Work out the finished part from the listing and answer in its coordinate system (mm). A direction names the side the tool comes from. Give positions to 0.01 mm unless a question says otherwise; leave off trailing zeros. Order: outer loops, then holes, each group sorted by start corner. A loop starts at its lowest first (then second) coordinate and runs counter-clockwise, first axis right, second up.
```python
from build123d import *

# Parameters (mm, degrees)
F0_R          = 25
F1_DEPTH      = 372
F2_R          = 5
F4_DEPTH      = 25
F4_DEPTH_BACK = 397


with BuildPart() as f1:
    # F0 (on Front) → F1 (new body)
    with BuildSketch(Plane.XZ):
        Circle(F0_R)
    extrude(amount=F1_DEPTH)

    # F2
    f2_edges = [f1.edges().sort_by_distance(p)[0] for p in [
        (-25, -372, 0),
        (-25, 0, 0),
    ]]
    fillet(f2_edges, radius=F2_R)

    # F3 (on face) → F4 (join, two sides)
    with BuildSketch(Plane(origin=(0, 0, 0), x_dir=(-1, 0, 0), z_dir=(0, 1, 0))) as f4_sk:
        Polygon((-0.001922, -6), (5.195191, -3.001664), (5.197113, 2.998336), (0.001922, 6), (-5.195191, 3.001664), (-5.197113, -2.998336), align=None)
    extrude(amount=F4_DEPTH)
    extrude(f4_sk.sketch, amount=-F4_DEPTH_BACK)


solid = f1.part
```
1. Straight lines are drawn through the part: probe 1 along X at (y, z) = (-31.5, 1.5); probe 2 along Y at (x, z) = (14, -12); probe 3 along Z at (x, y) = (1, -219.5). For each, find the intervals that lie inside material, in ascending order.
Findings below:
probe 1: x = -24.95 to 24.95
probe 2: y = -372 to 0
probe 3: z = -24.98 to 24.98
2. Which of the six approach directions +Z, -Z, +X, -X, +Y, -Y give full straight-line access (tool end or side, diameter ignored) to faces 1 (the face through (0, 25, 0)), 2 (the face through (4, -372, -4)), 3 (the face through (4, 0, -4))?
Findings below:
face 1: +Z, -Z, +X, -X, +Y
face 2: -Y
face 3: +Y
3. The part is cut by section A-A (y = -319). Write down the section's boundary in (x, z).
Findings below:
outline: circle Ø50 at (0, 0)
4. Given P1, Ø5, axis at x = 2, y = -227.5, coming from the +Z side; P2, Ø3, axis at y = -379, z = -0.5, coming from the -X side; P3, Ø6, axis at x = 5.5, z = -1, coming from the -Y side; P4, Ø5, axis at x = -12.5, y = -215.5, coming from the +Z side, each flat-ended and moving along its own axis, determine where each tip first touches the part or whether it passes through.
Findings below:
P1: stops at z = 25
P2: stops at x = -5.2
P3: stops at y = -397
P4: stops at z = 22.91
